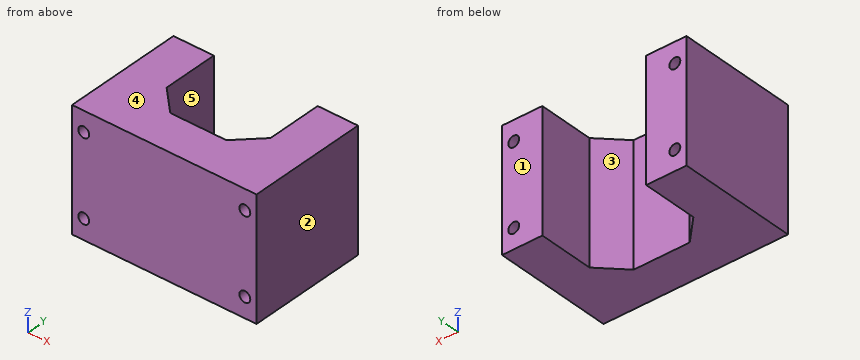
Autodesk Inventor part; units mm, degrees
ref_plane "Plano de trabajo1" through (0, -0.4184, 0) normal (0, 0, 1) x (1, 0, 0)
ref_plane "YZ Plane" through (0, 0, 0) normal (1, 0, 0) x (0, 1, 0)
ref_plane "XZ Plane" through (0, 0, 0) normal (0, 1, 0) x (-1, 0, 0)
ref_plane "Plano de trabajo1" through (0, -0.4184, 0) normal (0, 0, 1) x (1, 0, 0)
sketch "Boceto1" plane through (0, -0.4184, 0) normal (0, 0, 1) x (1, 0, 0)
  line L0 (51.8, 12.5012) -> (51.8, 40.2184)
  line L1 (51.8, 40.2184) -> (0.2, 40.2184)
  line L2 (0.2, 40.2184) -> (0.2, 12.5012)
  line L3 (0.2, 12.5012) -> (12.0828, 0.6184)
  line L4 (12.0828, 0.6184) -> (39.9172, 0.6184)
  line L5 (39.9172, 0.6184) -> (51.8, 12.5012)
  circle A0 centre (26, 20.4184) radius 14.2
  line L6 (71.8, 40.2184) -> (-19.8, 40.2184)
  line L7 (-19.8, 40.2184) -> (-19.8, -19.3816)
  line L8 (-19.8, -19.3816) -> (71.8, -19.3816)
  line L9 (71.8, -19.3816) -> (71.8, 40.2184)
  point P0 (0, 0.4184)
  point P1 (0.2, 40.2184)
  point P2 (51.8, 40.2184)
  dimension "d0" = 20
  dimension "d1" = 20
  dimension "d2" = 20
extrude "Extrusión1" add sketch "Boceto1" against normal blind 40 contours L0 L6 L9 L8 L7 L2 L3 L4 L5
sketch "Boceto2" plane through (0, -0.4184, 0) normal (0, 0, 1) x (1, 0, 0)
  line L0 (39.9172, 0.6184) -> (12.0828, 0.6184)
  line L1 (12.0828, 0.6184) -> (0.2, 12.5012)
  line L2 (0.2, 12.5012) -> (0.2, 40.2184)
  line L3 (0.2, 40.2184) -> (-19.8, 40.2184)
  line L4 (-19.8, 40.2184) -> (-19.8, -19.3816)
  line L5 (-19.8, -19.3816) -> (71.8, -19.3816)
  line L6 (71.8, -19.3816) -> (71.8, 40.2184)
  line L7 (71.8, 40.2184) -> (51.8, 40.2184)
  line L8 (51.8, 40.2184) -> (51.8, 12.5012)
  line L9 (51.8, 12.5012) -> (39.9172, 0.6184)
  point P0 (0, 0.4184)
extrude "Extrusión2" add sketch "Boceto2" along normal blind 10 and the other way blind 50
sketch "Boceto3" plane through (-19.8, 39.8, -50) normal (0, 1, 0) x (1, 0, 0)
  circle A0 centre (5.8, -10) radius 2.7
  circle A1 centre (5.8, -50) radius 2.7
  circle A2 centre (85.8, -10) radius 2.7
  circle A3 centre (85.8, -50) radius 2.7
  line L0 (0, 0) -> (20, 0)
  line L1 (59.7172, -60) -> (31.8828, -60)
  line L2 (45.8, -60) -> (45.8, 0)
  point P0 (19.8, -50)
  dimension "d9" = 80
  dimension "d10" = 5.4
  dimension "d11" = 40
  dimension "d12" = 10
  dimension "d13" = 40
extrude "Extrusión3" cut sketch "Boceto3" against normal through all
properties part number "UpperJawsuuport"
Can you work these out from the model? Positions are in its coordinate system, mm. Face numbers are marked on the shaded views. A direction names the side the tool comes from. Coordinates: 2 decimals unless noted, no trailing zeros. Order: outer loops, then holes, each group sorted by start corner. A loop starts at its lowest first (then second) coordinate and runs counter-clockwise, first axis right, second up. Notation, with made-up numbers: M -25,28.25 L 10,28.25 A22 cw 10,51.25 Z; hole C -4,52.25 d9. An arc over 180 degrees is marked long. Write item = value, one per line.
(1) Suppose I cut it at D-D on y = -5. Please give me the cut outline in (x, z).
Results are:
outline = M -19.8,-50 L 71.8,-50 L 71.8,10 L -19.8,10 Z; hole C -14,-40 d5.4; hole C -14,0 d5.4; hole C 66,-40 d5.4; hole C 66,0 d5.4
(2) Suppose I cut it at C-C on z = -40. Please give me the cut outline in (x, y), plus the area to 3 significant figures.
Results are:
outline = M -19.8,-19.8 L -16.7,-19.8 L -16.7,39.8 L -19.8,39.8 Z; M -11.3,-19.8 L 63.3,-19.8 L 63.3,39.8 L 51.8,39.8 L 51.8,12.08 L 39.92,0.2 L 12.08,0.2 L 0.2,12.08 L 0.2,39.8 L -11.3,39.8 Z; M 68.7,-19.8 L 71.8,-19.8 L 71.8,39.8 L 68.7,39.8 Z
area = 2,910 mm2
(3) I need wall thicknesses on line 1 along Z through (x, y) = (-14, 25); line 2 along X through (y, z) = (-2, 0); line 3 along X through (y, z) = (22, 0). Which ranges of each line are inside material? Lowest first, please. Write a range as [from, to].
Results are:
line_1 = [-50, -42.7], [-37.3, -2.7], [2.7, 10]
line_2 = [-19.8, -16.7], [-11.3, 63.3], [68.7, 71.8]
line_3 = [-19.8, -16.7], [-11.3, 0.2], [51.8, 63.3], [68.7, 71.8]
(4) For the marked faces 4 and 5, which set-ups out of +Z, -Z, +X, -X, +Y, -Y let a thin tool reach every point of the face, with its end or its side?
Results are:
face_4 = +Z, +X, -X, +Y, -Y
face_5 = +Z, -Z, +Y
(5) Suppose I cut it at B-B on x = -14. Please give me the cut outline in (y, z).
Results are:
outline = M -19.8,-50 L 39.8,-50 L 39.8,-42.7 L -19.8,-42.7 Z; M -19.8,-37.3 L 39.8,-37.3 L 39.8,-2.7 L -19.8,-2.7 Z; M -19.8,2.7 L 39.8,2.7 L 39.8,10 L -19.8,10 Z
(6) Suppose I cut it at A-A on y = 20. Please give me the cut outline in (x, z), plus the area to 3 significant figures.
Results are:
outline = M -19.8,-50 L 0.2,-50 L 0.2,10 L -19.8,10 Z; M 51.8,-50 L 71.8,-50 L 71.8,10 L 51.8,10 Z; hole C -14,-40 d5.4; hole C -14,0 d5.4; hole C 66,-40 d5.4; hole C 66,0 d5.4
area = 2,310 mm2
(7) For pin 1 Ø22.5 at (x, z) = (25.5, -29) entering from +Y; pin 2 Ø3 at (x, z) = (10, -9) entering from +Y, each with a flat end and sliding along its axis, tell me the tip position at first contact or that it passes through.
Results are:
pin_1 = 0.2
pin_2 = 3.78
(8) If we mould it in two halves opening along X, with no side actions, what happens to the marked faces 1, 2 and 3? For each: pulls with the +X half, pulls with the -X half, needs draft (parallel to the pull), parting line crosses it, or undercut.
Results are:
face_1 = needs draft
face_2 = pulls with the +X half
face_3 = undercut
